Geometry check sheet. Reference: the model listing, model coordinates, mm. A direction names the side the tool comes from. Round coordinates to 2 decimals unless told otherwise and drop trailing zeros. Write each loop counter-clockwise with the first axis right and the second up, starting at its lowest first coordinate (ties: lowest second). Pieces come first, ordered by that corner, then holes.
Item 1: Cross-section at C-C (x = 3.5). Enter the section's corners in (y, z).
Item 2: Cross-section at B-B (z = -78.5). Enter the section's corners in (x, y).
Item 3: Cross-section at A-A (y = 24). Enter the section's corners in (x, z), then the cut area to 3 significant figures.
Item 4: Draft check along X on faces 1 (the face through (-68.289, 6.603, 24.954)), 2 (the face through (-1, 1.6, -17)), 3 (the face through (-45, 19, -96)), 4 (the face through (69.1, 19, -8)). Enter one of: pulls with the +X half, pulls with the -X half, needs draft (parallel to the pull), parting line crosses it, or undercut.
Item 5: Access from +Z, -Z, +X, -X, +Y, -Y to the whole of each face (thin tool, end or side, straight path). Record for faces 5 (the face through (67.5, 20, -8)), 6 (the face through (-46.6, 23, -96)).
Item 6: Cross-section at D-D (z = 19). Enter the section's corners in (x, y).
Item 7: Depth check by flat-ended pin: P1, Ø20.5, axis at y = 27, z = -98, coming from the -X side; P2, Ø0.5, axis at x = -2, y = 0.5, coming from the -Z side; P3, Ø1.3, axis at x = -46, z = -86.5, coming from the +Y side; P4, Ø4.5, axis at y = 19, z = -17.07, coming from the +X side. Enter the tip coordinate at first touch or a pass-through.
Item 8: Scan lines: probe 1 along Z at (x, y) = (-62.5, 0.4); probe 2 along X at (y, z) = (10.5, 5); probe 3 along Y at (x, z) = (-2, 4.5). Record each from-to range of solid material in increasing order.
from build123d import *

# Parameters (mm, degrees)
BOSS_EXTRUDE2_DEPTH            = 1.6
EDGE_FLANGE1_STRIP_W           = 8.198
EDGE_FLANGE1_STRIP_H           = 1.6
EDGE_FLANGE1_STRIP_CUT_DEPTH   = 100
EDGE_FLANGE1_STRIP_2_W         = 8.198
EDGE_FLANGE1_STRIP_2_H         = 1.6
EDGE_FLANGE1_STRIP_CUT_2_DEPTH = 75.5
EDGE_FLANGE1_STRIP_3_W         = 8.198
EDGE_FLANGE1_STRIP_3_H         = 1.6
EDGE_FLANGE1_STRIP_CUT_3_DEPTH = 75.5
EDGE_FLANGE1_STRIP_4_W         = 8.198
EDGE_FLANGE1_STRIP_4_H         = 1.6
EDGE_FLANGE1_STRIP_CUT_4_DEPTH = 100
EDGE_FLANGE1_DEPTH             = 100
EDGE_FLANGE1_BEND_DEPTH        = 75.5
EDGE_FLANGE1_BEND_2_DEPTH      = 75.5
EDGE_FLANGE1_BEND_3_DEPTH      = 100
CUT_EXTRUDE1_START             = -69.018571159
CUT_EXTRUDE1_DEPTH             = 21.5
SKETCH24_R                     = 15
BOSS_EXTRUDE3_DEPTH            = 1.6
BOSS_EXTRUDE4_START            = -1.6
SKETCH25_R                     = 15
BOSS_EXTRUDE4_DEPTH            = 1.6
CUT_EXTRUDE2_DEPTH             = 109.6
CUT_EXTRUDE3_DEPTH             = 1000
M3_CLEARANCE_HOLE1_D           = 3.2
HOLE1_D                        = 3.4
HOLE1_DEPTH                    = 67.5
HOLE1_CBORE_D                  = 6
HOLE1_CBORE_DEPTH              = 16
CUT_EXTRUDE4_REACH             = 180.195
SKETCH36_R                     = 1.7


# Read off the part's stored shape, not the designer's step: Cut-Extrude1
# Sheet-metal steps are written as plain solids
with BuildPart() as part:
    # Sketch1 → Boss-Extrude2 (new body)
    with BuildSketch(Plane(origin=(0, 0, 0), x_dir=(1, 0, 0), z_dir=(0, 1, 0))):
        Polygon((45, 47.518571159), (45, 123.018571159), (30, 123.018571159), (30, 80.518571159), (-30, 80.518571159), (-30, 123.018571159), (-45, 123.018571159), (-45, 47.518571159), (-67.5, 47.518571159), (-67.5, -52.481428841), (67.5, -52.481428841), (67.5, 47.518571159), align=None)
    extrude(amount=BOSS_EXTRUDE2_DEPTH)

    # Edge-Flange1 strip (across the edge) → Edge-Flange1 strip cut (cut)
    with BuildSketch(Plane(origin=(-67.5, 1.6, -47.518571159), x_dir=(1, 0, 0), z_dir=(0, 0, 1))):
        with Locations((-3.2, -0.8)):
            Rectangle(EDGE_FLANGE1_STRIP_W, EDGE_FLANGE1_STRIP_H)
    extrude(amount=EDGE_FLANGE1_STRIP_CUT_DEPTH, mode=Mode.SUBTRACT)

    # Edge-Flange1 strip 2 (across the edge) → Edge-Flange1 strip cut 2 (cut)
    with BuildSketch(Plane(origin=(-45, 1.6, -123.018571159), x_dir=(1, 0, 0), z_dir=(0, 0, 1))):
        with Locations((-3.2, -0.8)):
            Rectangle(EDGE_FLANGE1_STRIP_2_W, EDGE_FLANGE1_STRIP_2_H)
    extrude(amount=EDGE_FLANGE1_STRIP_CUT_2_DEPTH, mode=Mode.SUBTRACT)

    # Edge-Flange1 strip 3 (across the edge) → Edge-Flange1 strip cut 3 (cut)
    with BuildSketch(Plane(origin=(45, 1.6, -47.518571159), x_dir=(-1, 0, 0), z_dir=(0, 0, -1))):
        with Locations((-3.2, -0.8)):
            Rectangle(EDGE_FLANGE1_STRIP_3_W, EDGE_FLANGE1_STRIP_3_H)
    extrude(amount=EDGE_FLANGE1_STRIP_CUT_3_DEPTH, mode=Mode.SUBTRACT)

    # Edge-Flange1 strip 4 (across the edge) → Edge-Flange1 strip cut 4 (cut)
    with BuildSketch(Plane(origin=(67.5, 1.6, 52.481428841), x_dir=(-1, 0, 0), z_dir=(0, 0, -1))):
        with Locations((-3.2, -0.8)):
            Rectangle(EDGE_FLANGE1_STRIP_4_W, EDGE_FLANGE1_STRIP_4_H)
    extrude(amount=EDGE_FLANGE1_STRIP_CUT_4_DEPTH, mode=Mode.SUBTRACT)

    # Edge-Flange1 section (across the edge) → Edge-Flange1 (add)
    with BuildSketch(Plane(origin=(-67.5, 1.6, -47.518571159), x_dir=(1, 0, 0), z_dir=(0, 0, 1))):
        with BuildLine():
            Line((-1.6, 0.899), (-1.6, 35))
            Line((-1.6, 35), (0, 35))
            Line((0, 35), (0, 0.899))
            ThreePointArc((0, 0.899), (0.263311004, 0.263311004), (0.899, 0))
            Line((0.899, 0), (0.899, -1.6))
            ThreePointArc((0.899, -1.6), (-0.868059846, -0.868059846), (-1.6, 0.899))
        make_face()
    extrude(amount=EDGE_FLANGE1_DEPTH)

    # Edge-Flange1 section 2 (across the edge) → Edge-Flange1 bend (add)
    with BuildSketch(Plane(origin=(-45, 1.6, -123.018571159), x_dir=(1, 0, 0), z_dir=(0, 0, 1))):
        with BuildLine():
            Line((-1.6, 0.899), (-1.6, 35))
            Line((-1.6, 35), (0, 35))
            Line((0, 35), (0, 0.899))
            ThreePointArc((0, 0.899), (0.263311004, 0.263311004), (0.899, 0))
            Line((0.899, 0), (0.899, -1.6))
            ThreePointArc((0.899, -1.6), (-0.868059846, -0.868059846), (-1.6, 0.899))
        make_face()
    extrude(amount=EDGE_FLANGE1_BEND_DEPTH)

    # Edge-Flange1 section 3 (across the edge) → Edge-Flange1 bend 2 (add)
    with BuildSketch(Plane(origin=(45, 1.6, -47.518571159), x_dir=(-1, 0, 0), z_dir=(0, 0, -1))):
        with BuildLine():
            Line((-1.6, 0.899), (-1.6, 35))
            Line((-1.6, 35), (0, 35))
            Line((0, 35), (0, 0.899))
            ThreePointArc((0, 0.899), (0.263311004, 0.263311004), (0.899, 0))
            Line((0.899, 0), (0.899, -1.6))
            ThreePointArc((0.899, -1.6), (-0.868059846, -0.868059846), (-1.6, 0.899))
        make_face()
    extrude(amount=EDGE_FLANGE1_BEND_2_DEPTH)

    # Edge-Flange1 section 4 (across the edge) → Edge-Flange1 bend 3 (add)
    with BuildSketch(Plane(origin=(67.5, 1.6, 52.481428841), x_dir=(-1, 0, 0), z_dir=(0, 0, -1))):
        with BuildLine():
            Line((-1.6, 0.899), (-1.6, 35))
            Line((-1.6, 35), (0, 35))
            Line((0, 35), (0, 0.899))
            ThreePointArc((0, 0.899), (0.263311004, 0.263311004), (0.899, 0))
            Line((0.899, 0), (0.899, -1.6))
            ThreePointArc((0.899, -1.6), (-0.868059846, -0.868059846), (-1.6, 0.899))
        make_face()
    extrude(amount=EDGE_FLANGE1_BEND_3_DEPTH)

    # Cut-Extrude1 outline → Cut-Extrude1 (cut)
    with BuildSketch(Plane.XY.offset(CUT_EXTRUDE1_START)):
        with BuildLine():
            ThreePointArc((45, 2.499), (44.736688996, 1.863311004), (44.101, 1.6))
            Line((44.101, 1.6), (44.101, 0))
            ThreePointArc((44.101, 0), (45.868059846, 0.731940154), (46.6, 2.499))
            Line((46.6, 2.499), (46.6, 36.6))
            Line((46.6, 36.6), (45, 36.6))
            Line((45, 36.6), (45, 2.499))
        make_face()
        with BuildLine():
            ThreePointArc((-46.6, 2.499), (-45.868059846, 0.731940154), (-44.101, 0))
            Line((-44.101, 0), (-44.101, 1.6))
            ThreePointArc((-44.101, 1.6), (-44.736688996, 1.863311004), (-45, 2.499))
            Line((-45, 2.499), (-45, 36.6))
            Line((-45, 36.6), (-46.6, 36.6))
            Line((-46.6, 36.6), (-46.6, 2.499))
        make_face()
    extrude(amount=CUT_EXTRUDE1_DEPTH, mode=Mode.SUBTRACT)

    # Sketch24 → Boss-Extrude3 (add)
    with BuildSketch(Plane(origin=(46.6, 0, 0), x_dir=(0, 0, -1), z_dir=(1, 0, 0))):
        with Locations((108.018571159, 28.1)):
            Circle(SKETCH24_R)
    extrude(amount=-BOSS_EXTRUDE3_DEPTH)

    # Sketch25 → Boss-Extrude4 (add)
    with BuildSketch(Plane.ZY.offset(46.6).offset(BOSS_EXTRUDE4_START)):
        with Locations((-108.018571159, 28.1)):
            Circle(SKETCH25_R)
    extrude(amount=BOSS_EXTRUDE4_DEPTH)

    # Sketch26 → Cut-Extrude2 (cut)
    with BuildSketch(Plane(origin=(46.6, 0, 0), x_dir=(0, 0, -1), z_dir=(1, 0, 0))):
        with BuildLine():
            Line((120.377778253, 36.6), (123.018571159, 36.6))
            Line((123.018571159, 36.6), (123.018571159, 28.1))
            ThreePointArc((123.018571159, 28.1), (122.343167251, 32.550387263), (120.377778253, 36.6))
        make_face()
    extrude(amount=-CUT_EXTRUDE2_DEPTH, mode=Mode.SUBTRACT)

    # Sketch27 → Cut-Extrude3 (cut)
    with BuildSketch(Plane(origin=(69.1, 0, 0), x_dir=(0, 0, -1), z_dir=(1, 0, 0))):
        with BuildLine():
            Line((-37.729365474, 19.100000095), (-37.729365474, 36.6))
            Line((-37.729365474, 36.6), (-12.729365474, 36.6))
            Line((-12.729365474, 36.6), (-12.729365474, 19.100000095))
            ThreePointArc((-12.729365474, 19.100000095), (-25.229365474, 6.600000095), (-37.729365474, 19.100000095))
        make_face()
    extrude(amount=-CUT_EXTRUDE3_DEPTH, mode=Mode.SUBTRACT)

    # M3 Clearance Hole1 (through all)
    with Locations(Plane(origin=(0, 1.6, -32.518571159), x_dir=(-1, 0, 0), z_dir=(0, 1, 0))):
        with Locations((-62.5, -11.814648696), (62.5, -11.814648696), (62.5, 80), (-62.5, 80), (-37.5, -57.632792906), (37.5, -57.632792906)):
            Hole(M3_CLEARANCE_HOLE1_D / 2)

    # Hole1
    with Locations(Plane(origin=(120, 6.6, -32.518571159), x_dir=(0, 0, 1), z_dir=(1, 0, 0))):
        with Locations((15.451100734, -12.39688985)):
            hole1 = CounterBoreHole(HOLE1_D / 2, HOLE1_CBORE_D / 2, HOLE1_CBORE_DEPTH, depth=HOLE1_DEPTH)

    # Mirror1: Hole1 across Right Plane
    add(hole1.mirror(Plane(origin=(0, 0, 0), x_dir=(0, 0, -1), z_dir=(1, 0, 0))), mode=Mode.SUBTRACT)

    # Sketch36 → Cut-Extrude4 (cut, up to next)
    with BuildSketch(Plane(origin=(-80, 6.6, -32.518571159), x_dir=(0, 0, 1), z_dir=(-1, 0, 0)), mode=Mode.PRIVATE) as cut_extrude4_sk1:
        with Locations(Location((-53.294944095, 8.283400622, 0), (0, 0, 90))):
            Circle(SKETCH36_R)
    cut_extrude4_tool1 = extrude(cut_extrude4_sk1.sketch, amount=-CUT_EXTRUDE4_REACH, mode=Mode.PRIVATE) & part.part
    add(cut_extrude4_tool1.solids().sort_by_distance((-80, 14.883401, -85.813515))[0], mode=Mode.SUBTRACT)


solid = part.part
Resolved:
1. outline: (0, -80.52) - (1.6, -80.52) - (1.6, 52.48) - (0, 52.48) - close
2. outline: (-46.6, 2.5) arc R2.5 ccw to (-44.1, 0) - (44.1, 0) arc R2.5 ccw to (46.6, 2.5) - (46.6, 36.6) - (45, 36.6) - (45, 2.5) arc R0.9 cw to (44.1, 1.6) - (-44.1, 1.6) arc R0.9 cw to (-45, 2.5) - (-45, 36.6) - (-46.6, 36.6) - close
3. outline: (-69.1, -47.52) - (-67.5, -47.52) - (-67.5, 12.73) - (-69.1, 12.73) - close; (-69.1, 37.73) - (-67.5, 37.73) - (-67.5, 52.48) - (-69.1, 52.48) - close; (-46.6, -123.02) - (-45, -123.02) - (-45, -69.02) - (-46.6, -69.02) - close; (45, -123.02) - (46.6, -123.02) - (46.6, -69.02) - (45, -69.02) - close; (67.5, -47.52) - (69.1, -47.52) - (69.1, 12.73) - (67.5, 12.73) - close; (67.5, 37.73) - (69.1, 37.73) - (69.1, 52.48) - (67.5, 52.48) - close
3. area: 413 mm2
4. face 1: needs draft
4. face 2: undercut
4. face 3: undercut
4. face 4: pulls with the +X half
5. face 5: +Z, -Z, +Y
5. face 6: +Z, -Z, -X, +Y, -Y
6. outline: (-69.1, 2.5) arc R2.5 ccw to (-66.6, 0) - (66.6, 0) arc R2.5 ccw to (69.1, 2.5) - (69.1, 8.26) - (67.5, 8.26) - (67.5, 2.5) arc R0.9 cw to (66.6, 1.6) - (-66.6, 1.6) arc R0.9 cw to (-67.5, 2.5) - (-67.5, 8.26) - (-69.1, 8.26) - close
7. P1: stops at x = -46.6
7. P2: stops at z = -80.52
7. P3: stops at y = 36.6
7. P4: stops at x = 69.1
8. probe 1: z = -47.52 to -45.93, -42.73 to 45.88, 49.08 to 52.48
8. probe 2: x = -69.1 to -67.5, 67.5 to 69.1
8. probe 3: y = 0 to 1.6
